from build123d import *

# Parameters (mm, degrees)
SKETCH1_R           = 75
BOSS_EXTRUDE1_DEPTH = 10
BOSS_EXTRUDE2_DEPTH = 10
SKETCH3_R           = 2.5
SKETCH3_R_2         = 3.75
CUT_EXTRUDE1_DEPTH  = 144.351459106
CIRPATTERN1_COUNT   = 4
CUT_EXTRUDE2_START  = -5
SKETCH4_R           = 5.043629395
CUT_EXTRUDE2_DEPTH  = 149.351459106
CIRPATTERN2_COUNT   = 4


with BuildPart() as part:
    # Sketch1 → Boss-Extrude1 (new body)
    with BuildSketch(Plane.YZ):
        with Locations(Location((0, 0, 0), (0, 0, 270))):
            Circle(SKETCH1_R)
    extrude(amount=BOSS_EXTRUDE1_DEPTH)

    # Sketch2 → Boss-Extrude2 (add)
    with BuildSketch(Plane(origin=(0, 0, 0), x_dir=(0, -1, 0), z_dir=(-1, 0, 0))):
        with BuildLine():
            Line((-92.771012238, 7.974028306), (92.382035247, 7.974028306))
            ThreePointArc((92.382035247, 7.974028306), (100.356063553, 0), (92.382035247, -7.974028306))
            Line((92.382035247, -7.974028306), (-92.771012238, -7.974028306))
            ThreePointArc((-92.771012238, -7.974028306), (-100.745040543, 0), (-92.771012238, 7.974028306))
        make_face()
        with BuildLine():
            Line((-7.968256638, -92.769682141), (-7.968256638, 93.521041486))
            ThreePointArc((-7.968256638, 93.521041486), (0, 101.489298124), (7.968256638, 93.521041486))
            Line((7.968256638, 93.521041486), (7.968256638, -92.769682141))
            ThreePointArc((7.968256638, -92.769682141), (0, -100.73793878), (-7.968256638, -92.769682141))
        make_face()
    extrude(amount=-BOSS_EXTRUDE2_DEPTH)

    # Sketch3 → Cut-Extrude1 (cut, symmetric)
    with BuildSketch(Plane.YZ.offset(10)):
        with Locations(Location((0, 70, 0), (0, 0, 270))):
            Circle(SKETCH3_R)
        with Locations(Location((0, 93.46793349, 0), (0, 0, 270))):
            Circle(SKETCH3_R_2)
    cut_extrude1 = extrude(amount=CUT_EXTRUDE1_DEPTH, both=True, mode=Mode.SUBTRACT)

    # CirPattern1: Cut-Extrude1 ×4 about axis
    cirpattern1_axis = Axis((0, 0.032009754, -0.225189286), (1, 0, 0))
    for i in range(1, CIRPATTERN1_COUNT):
        add(cut_extrude1.rotate(cirpattern1_axis, i * 360 / CIRPATTERN1_COUNT), mode=Mode.SUBTRACT)

    # Sketch4 → Cut-Extrude2 (cut)
    with BuildSketch(Plane.YZ.offset(10).offset(CUT_EXTRUDE2_START)):
        with Locations(Location((0, 70, 0), (0, 0, 90))):
            Circle(SKETCH4_R)
    cut_extrude2 = extrude(amount=CUT_EXTRUDE2_DEPTH, mode=Mode.SUBTRACT)

    # CirPattern2: Cut-Extrude2 ×4 about axis
    cirpattern2_axis = Axis((0, 0.032003773, -0.157220476), (1, 0, 0))
    for i in range(1, CIRPATTERN2_COUNT):
        add(cut_extrude2.rotate(cirpattern2_axis, i * 360 / CIRPATTERN2_COUNT), mode=Mode.SUBTRACT)


solid = part.part
Read the model definition and answer for the solid it produces. Units are mm, in the model's axes. A direction names the side the tool comes from. Give positions to 0.01 mm unless a question says otherwise; leave off trailing zeros. Loops run counter-clockwise (first coordinate to the right, second up) from the corner with the lowest first, then second, coordinate; pieces in that order, holes last. Notation, with made-up numbers: (89.25, 63) -> (99.25, 63) arc R24 cw to (99.25, 95) -> close; hole circle Ø10 at (20.25, 7). An arc over 180 degrees is marked (long way). Answer as CSV lines item,"result".
Item 1: For faces 1 (the face through (5, -83, 7.974)), 2 (the face through (5, 7.968, 84)), 3 (the face through (5, -67.8, 0.9)), 4 (the face through (5, -84, -7.974)), 5 (the face through (4.93, -0.175, -100.736)), determine the directions among +Z, -Z, +X, -X, +Y, -Y from which every point of the face is accessible in a straight line to the end or side of a thin tool.
Returned:
face 1,"+Z, +X, -X, -Y"
face 2,"+Z, +X, -X, +Y"
face 3,"+X"
face 4,"-Z, +X, -X, -Y"
face 5,"-Z, +X, -X"
Item 2: Determine the mould class of faces 6 (the face through (0, -1, 2)), 7 (the face through (4.93, 53.53, 52.53)), 8 (the face through (5, 69, 2.2)) for opening direction Z: +Z half, -Z half, draft (parallel to the pull), parting line (faces both ways), or undercut.
Returned:
face 6,"draft"
face 7,"+Z half"
face 8,"undercut"
Item 3: Find section C-C on y = -13. Give the vertices of the cut face in (x, z), plus the area to 3 significant figures.
Returned:
outline,"(0, -73.86) -> (10, -73.86) -> (10, 73.86) -> (0, 73.86) -> close"
area,"1,480 mm²"
Item 4: Find section A-A on x = 1.75. State how many separate pieces and enclosed holes the cut face has, plus the area to 3 significant figures.
Returned:
separate pieces,"1"
enclosed holes,"8"
area,"19,000 mm²"
Item 5: Each of these flat-tipped pins is pushed along its axis until it touches: pin 1 (16 mm diameter, centred on y = -70.13, z = -0.19, fed in from -X); pin 2 (3 mm diameter, centred on x = 6.5, z = 85, fed in from -Y); pin 3 (6 mm diameter, centred on x = 4, z = 27.5, fed in from -Y); pin 4 (8 mm diameter, centred on y = 0, z = 70, fed in from +X). Where does it stop, or does it pass through?
Returned:
pin 1,"stops at x = 0"
pin 2,"stops at y = -7.97"
pin 3,"stops at y = -70.89"
pin 4,"stops at x = 5"
Item 6: Consider line 1 (X direction, y = 72.5, z = -2.5); line 2 (Y direction, x = 6.5, z = -86.5). Determine where each line is inside the solid, lowest interval first. Write a range as [from, to].
Returned:
line 1,"x = [0, 5]"
line 2,"y = [-7.97, 7.97]"
Item 7: Find section B-B on z = 43.5. Give the vertices of the cut face in (x, y).
Returned:
outline,"(0, -61.1) -> (10, -61.1) -> (10, 61.1) -> (0, 61.1) -> close"
